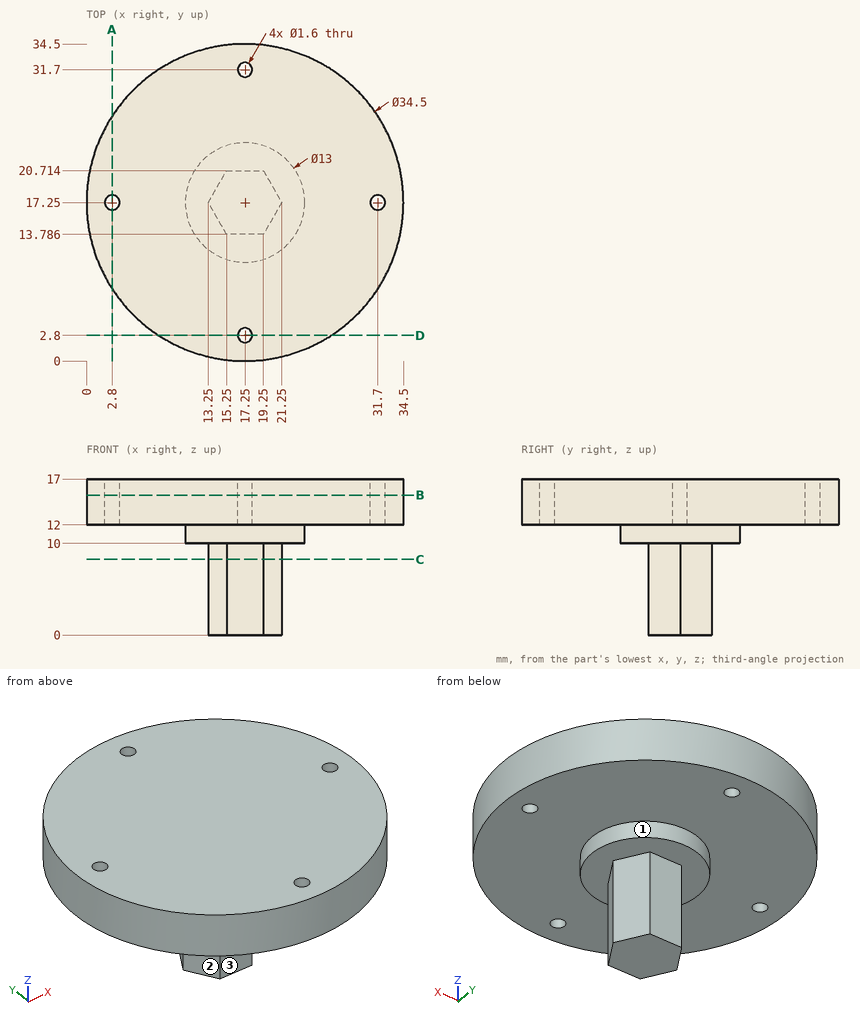
Check sheet for the drawn part. Datum: minimum x, y, z corner. Units: mm. A direction names the side the tool comes from. Round coordinates to 2 decimals unless told otherwise and drop trailing zeros. Order: outer loops, then holes, each group sorted by start corner. A loop starts at its lowest first (then second) coordinate and runs counter-clockwise, first axis right, second up.
(1) Scan lines: probe 1 along Y at (x, z) = (17.25, 15); probe 2 along Z at (x, y) = (15, 20.5); probe 3 along X at (y, z) = (2.8, 14.3). Record each from-to range of solid material in increasing order.
(2) Cross-section at B-B, the plane z = 15.25. Enter the section's corners in (x, y), and give its area (3 significant figures).
(3) Go/stop test with flat-tipped pins: P1, Ø2, axis at x = 16.5, z = 5, coming from the -Y side; P2, Ø2, axis at x = 16.5, z = 4, coming from the +Y side; P3, Ø3, axis at x = 30, z = 15, coming from the +Y side. Record where each tip stops, or that it passes through.
(4) Cross-section at A-A, the plane x = 2.8. Enter the section's corners in (y, z), and give its area (3 significant figures).
(5) Access from +Z, -Z, +X, -X, +Y, -Y to the whole of each face (thin tool, end or side, straight path). Record for the marked faces 1, 2 and 3.
(6) Cross-section at C-C, the plane z = 8.25. Enter the section's corners in (x, y).
Check sheet entries:
1. probe 1: y = 0 to 2, 3.6 to 30.9, 32.5 to 34.5
1. probe 2: z = 10 to 17
1. probe 3: x = 7.83 to 16.45, 18.05 to 26.67
2. outline: circle Ø34.5 at (17.25, 17.25); hole circle Ø1.6 at (2.8, 17.25); hole circle Ø1.6 at (17.25, 2.8); hole circle Ø1.6 at (17.25, 31.7); hole circle Ø1.6 at (31.7, 17.25)
2. area: 927 mm2
3. P1: stops at y = 13.79
3. P2: stops at y = 20.71
3. P3: stops at y = 30.33
4. outline: (7.83, 12) - (16.45, 12) - (16.45, 17) - (7.83, 17) - close; (18.05, 12) - (26.67, 12) - (26.67, 17) - (18.05, 17) - close
4. area: 86.2 mm2
5. face 1: -Z
5. face 2: -Z, -X, -Y
5. face 3: -Z, +X, -X, -Y
6. outline: (13.25, 17.25) - (15.25, 13.79) - (19.25, 13.79) - (21.25, 17.25) - (19.25, 20.71) - (15.25, 20.71) - close
